from build123d import *

# Parameters (mm, degrees)
CUT_EXTRUDE2_START = 18
CUT_EXTRUDE2_DEPTH = 5.2
SKETCH4_R          = 3
CUT_EXTRUDE3_DEPTH = 20


with BuildPart() as part:
    # Sketch1 → Revolve1 (revolve)
    with BuildSketch(Plane.XY, mode=Mode.PRIVATE) as revolve1_sk:
        with BuildLine():
            Line((-4.185051691, 0), (-4.185051691, 11.5))
            Line((-4.185051691, 11.5), (-3.185051691, 12.5))
            Line((-3.185051691, 12.5), (-0.484378869, 12.5))
            Line((-0.484378869, 12.5), (-0.484378869, 11.45))
            Line((-0.484378869, 11.45), (0.815621131, 11.45))
            Line((0.815621131, 11.45), (0.815621131, 12.5))
            Line((0.815621131, 12.5), (17.814948309, 12.5))
            Line((17.814948309, 12.5), (17.814948309, 17.5))
            Line((17.814948309, 17.5), (27.814948309, 17.5))
            Line((27.814948309, 17.5), (27.814948309, 21))
            Line((27.814948309, 21), (37.814948309, 21))
            Line((37.814948309, 21), (37.814948309, 17.5))
            Line((37.814948309, 17.5), (87.814948309, 17.5))
            Line((87.814948309, 17.5), (87.916312777, 16.636677786))
            ThreePointArc((87.916312777, 16.636677786), (87.982028112, 16.510560309), (88.114948309, 16.46))
            Line((88.114948309, 16.46), (89.414948309, 16.46))
            ThreePointArc((89.414948309, 16.46), (89.978347351, 16.823399043), (89.614948309, 17.386798085))
            Line((89.614948309, 17.386798085), (89.614948309, 18.226798085))
            Line((89.614948309, 18.226798085), (130.114948309, 18.226798085))
            Line((130.114948309, 18.226798085), (130.114948309, 15.726798085))
            Line((130.114948309, 15.726798085), (147.114948309, 15.726798085))
            Line((147.114948309, 15.726798085), (147.114948309, 11.45))
            Line((147.114948309, 11.45), (148.414948309, 11.45))
            Line((148.414948309, 11.45), (148.414948309, 12.5))
            Line((148.414948309, 12.5), (247.114948309, 12.5))
            Line((247.114948309, 12.5), (248.114948309, 11.5))
            Line((248.114948309, 11.5), (248.114948309, 0))
            Line((248.114948309, 0), (-4.185051691, 0))
        make_face()
    revolve(revolve1_sk.sketch.rotate(Axis((-15.310878374, 0, 0), (1, 0, 0)), 180), axis=Axis((-15.310878374, 0, 0), (1, 0, 0)))

    # Sketch3 → Cut-Extrude2 (cut)
    with BuildSketch(Plane(origin=(0, 0, 0), x_dir=(1, 0, 0), z_dir=(0, 1, 0)).offset(CUT_EXTRUDE2_START)):
        with BuildLine():
            Line((51.814948309, 5), (73.814948309, 5))
            ThreePointArc((73.814948309, 5), (78.814948309, 0), (73.814948309, -5))
            Line((73.814948309, -5), (51.814948309, -5))
            ThreePointArc((51.814948309, -5), (46.814948309, 0), (51.814948309, 5))
        make_face()
    extrude(amount=-CUT_EXTRUDE2_DEPTH, mode=Mode.SUBTRACT)

    # Sketch4 → Cut-Extrude3 (cut, symmetric)
    with BuildSketch(Plane(origin=(0, 0, 0), x_dir=(1, 0, 0), z_dir=(0, 1, 0))):
        with Locations(Location((233.114948309, 0, 0), (0, 0, 270))):
            Circle(SKETCH4_R)
    extrude(amount=CUT_EXTRUDE3_DEPTH, both=True, mode=Mode.SUBTRACT)


solid = part.part
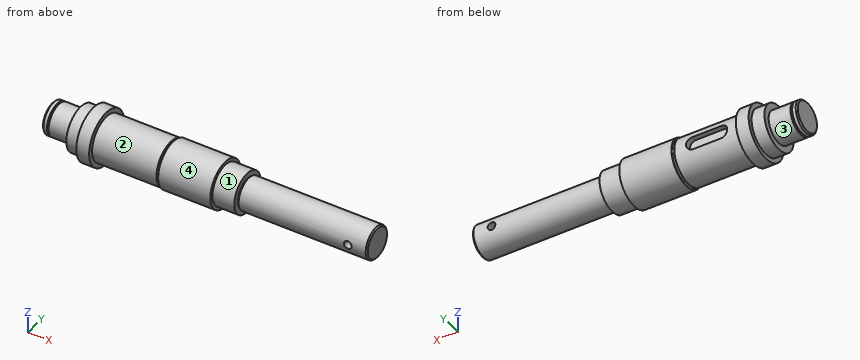
The listing builds one solid part. Answer for the finished solid, in the listing's coordinates (mm). Face numbers are marked on the shaded views. A direction names the side the tool comes from. Coordinates: 2 decimals unless noted, no trailing zeros. Loops run counter-clockwise (first coordinate to the right, second up) from the corner with the lowest first, then second, coordinate; pieces in that order, holes last. Notation, with made-up numbers: (-4.75, 46) -> (6.25, 46) arc R33 ccw to (6.25, 77) -> close; hole circle Ø4 at (31.5, 20.25). An arc over 180 degrees is marked (long way). Write item = value, one per line. Start each with the question number.
1) A cutting plane is placed at A-A (x = 162). Give the vertices of the cut face in (y, z), then the cut area to 3 significant figures.
2) Given pin 1 Ø3 at (x, y) = (68.5, 14) entering from -Z; pin 2 Ø8 at (x, z) = (69, 0.5) entering from +Y; pin 3 Ø8 at (x, y) = (93.5, -6.5) entering from -Z, each flat-ended and moving along its own axis, determine where each tip first touches the part or whether it passes through.
3) A tool of negligible diameter and unlimited length cuts with its end or side. For the marked faces 3 and 4, from which of +Z, -Z, +X, -X, +Y, -Y can it reach the whole face along a straight path? Write none if from no direction.
4) Straight lines are drawn through the part: line 1 (X direction, y = -12, z = -4.5); line 2 (X direction, y = 7.25, z = 0); line 3 (Z direction, x = 81, y = -1.5). For each, find the intervals that lie inside material, in ascending order. Write a range as from..to.
5) The mould has two halves that part along X. Classify the marked faces 1 and 2: released by +X, released by -X, zero draft, split by the parting line, or undercut.
Responses:
q1.outline = circle Ø25 at (0, 0)
q1.area = 491 mm²
q2.pin_1 = -12.25
q2.pin_2 = 12.8
q2.pin_3 = -18.05
q3.face_3 = -X
q3.face_4 = +X
q4.line_1 = 17.81..147.11
q4.line_2 = -4.19..230.11, 236.11..248.11
q4.line_3 = -17.44..17.44
q5.face_1 = zero draft
q5.face_2 = undercut
